The figure shows three views and two pictorial views of one solid part (mm, origin at its lowest corner). Answer the questions. Coordinates: 2 decimals unless noted, no trailing zeros. Loops run counter-clockwise (first coordinate to the right, second up) from the corner with the lowest first, then second, coordinate; pieces in that order, holes last. Notation, with made-up numbers: M 29.5,59.5 L 58.5,59.5 A20 ccw 58.5,86.5 Z; hole C -28,86.25 d10. An arc over 180 degrees is marked long. Answer as a JSON object with one key per item and string values. Group by question number.
1. A cutting plane is placed at A-A on z = 3. Give the vertices of the cut face in (x, y).
2. A cutting plane is placed at C-C on y = 2.5. Give the vertices of the cut face in (x, z), and give its area (3 significant figures).
3. A straight line is drawn through the part: L1, parallel to X at y = 0.45, z = 5.5. Find the intervals that lie inside material, in ascending order.
4. Given pin 1 (0.9 mm diameter, centred on y = 1.5, z = 4, fed in from -X), flat-ended and moving along its own axis, determine where the tip first touches the part or whether it passes through.
5. A cutting plane is placed at B-B on y = 0.3. Give the vertices of the cut face in (x, z), and give its area (3 significant figures).
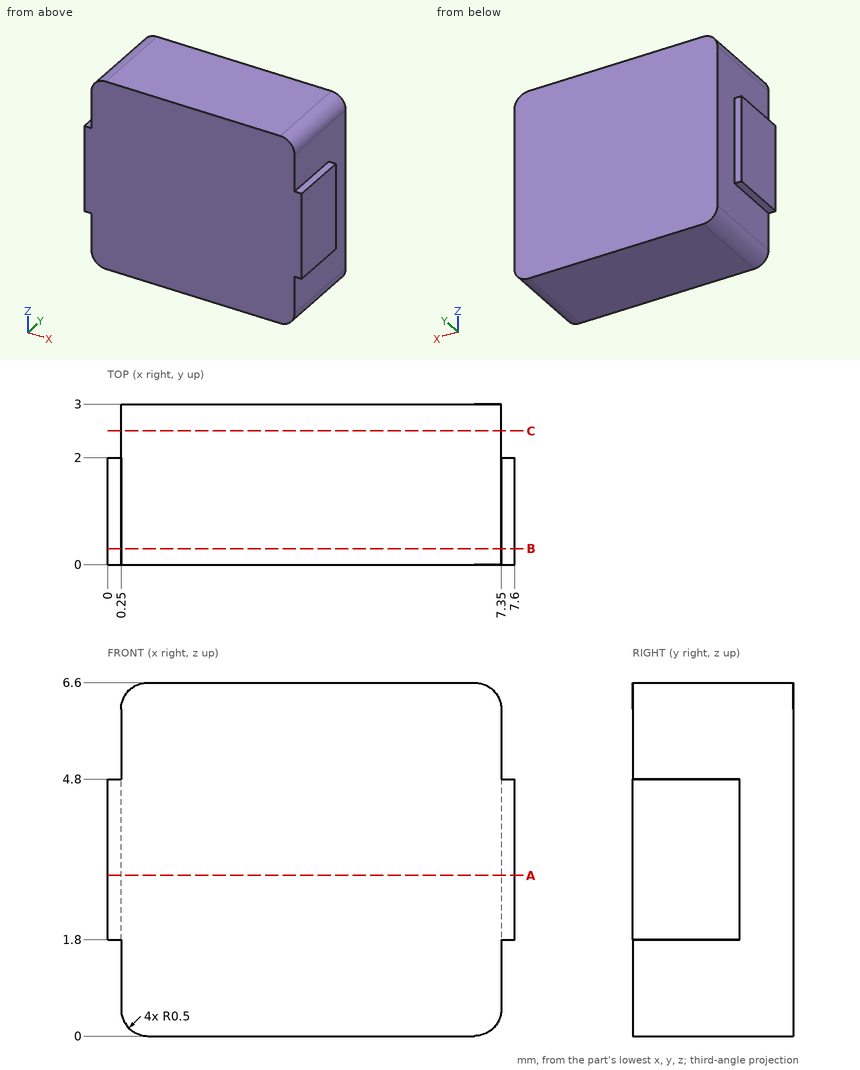
From the geometry:
{
 "1": {"outline": "M 0,0 L 7.6,0 L 7.6,2 L 7.35,2 L 7.35,3 L 0.25,3 L 0.25,2 L 0,2 Z"},
 "2": {"outline": "M 0.25,0.5 A0.5 ccw 0.75,0 L 6.85,0 A0.5 ccw 7.35,0.5 L 7.35,6.1 A0.5 ccw 6.85,6.6 L 0.75,6.6 A0.5 ccw 0.25,6.1 Z", "area": "46.6 mm²"},
 "3": {"L1": "x = 0.25 to 7.35"},
 "4": {"pin 1": "stops at x = 0"},
 "5": {"outline": "M 0,1.8 L 0.25,1.8 L 0.25,0.5 A0.5 ccw 0.75,0 L 6.85,0 A0.5 ccw 7.35,0.5 L 7.35,1.8 L 7.6,1.8 L 7.6,4.8 L 7.35,4.8 L 7.35,6.1 A0.5 ccw 6.85,6.6 L 0.75,6.6 A0.5 ccw 0.25,6.1 L 0.25,4.8 L 0,4.8 Z", "area": "48.1 mm²"}
}
